For this review, take the finished solid that the model builds, in its own axes (mm). Face numbers are marked on the shaded views. A direction names the side the tool comes from. Give positions to 0.01 mm unless a question says otherwise; leave off trailing zeros. Order: outer loops, then holes, each group sorted by start corner. A loop starts at its lowest first (then second) coordinate and runs counter-clockwise, first axis right, second up. Notation, with made-up numbers: (-5, -27.5) - (26, -27.5) arc R22 ccw to (26, 1.5) - close; hole circle Ø11 at (-35, 40). An arc over 180 degrees is marked (long way). Use a Markdown table: item, result. Add a question column.
1) We need section C-C on y = 113. Write out the cut boundary in (x, z), then the cut area to 3 significant figures.
2) We need section B-B on y = 121.5. Write out the cut boundary in (x, z), then the cut area to 3 significant figures.
3) Wall thickness on L1, parallel to Z at x = -30.25, y = 115.5; L2, parallel to Z at x = -24.5, y = 112.5; L3, parallel to X at y = 127.25, z = 3: over which ranges is each line inside the solid? List them lowest first.
4) Clearance check with flat-ended pins moving along their axes: P1, Ø0.6, axis at y = 116, z = 2.5, coming from the +X side; P2, Ø1, axis at x = -31.5, y = 115, coming from the +Z side; P3, Ø1, axis at x = -23.5, z = 3, coming from the -Y side; P4, Ø3, axis at x = -32, y = 126.5, coming from the -Z side. State where each tip first meets the part, or that it passes through.
5) Machinability: for the marked faces 1, 2 and 3, which of the approach directions +Z, -Z, +X, -X, +Y, -Y give a long, thin tool a straight path to every point of the face, cutting with its end or side? Answer none if there is none.
6) We need section A-A on x = -33.25. Write out the cut boundary in (y, z), then the cut area to 3 significant figures.
7) We need section D-D on x = -27. Write out the cut boundary in (y, z) (3 decimals).
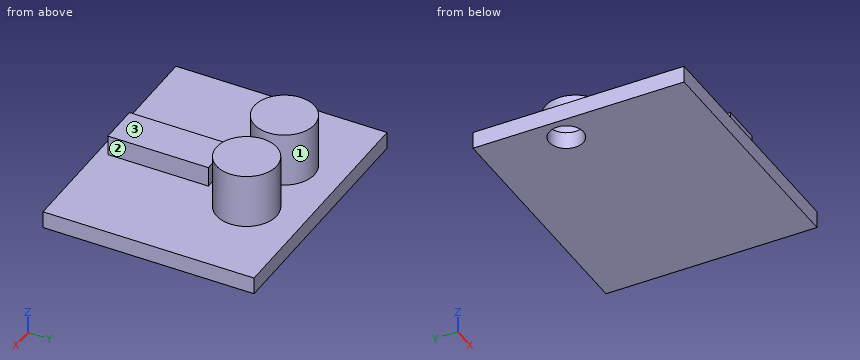
```python
from build123d import *

# Parameters (mm, degrees)
SKETCH_1_W      = 24.7
SKETCH_1_H      = 21
SKETCH_1_R      = 1.7
EXTRUDE_1_DEPTH = 1.7
SKETCH_2_R      = 3
EXTRUDE_2_DEPTH = 5.4
SKETCH_3_W      = 4
SKETCH_3_H      = 10
EXTRUDE_3_DEPTH = 2


with BuildPart() as part:
    # Эскиз1 → Бобышка-Вытянуть1 (new body)
    with BuildSketch(Plane.XY):
        with Locations((-24.007558734, 119.994849308)):
            Rectangle(SKETCH_1_W, SKETCH_1_H)
        with Locations((-33.957558734, 122.494849308)):
            Circle(SKETCH_1_R, mode=Mode.SUBTRACT)
    extrude(amount=EXTRUDE_1_DEPTH)

    # Эскиз2 → Бобышка-Вытянуть2 (add)
    with BuildSketch(Plane.XY.offset(1.7)):
        with Locations(Location((-27.825017342, 124.86066732, 0), (0, 0, 180))):
            Circle(SKETCH_2_R)
        with Locations(Location((-20.796714073, 124.86066732, 0), (0, 0, 180))):
            Circle(SKETCH_2_R)
    extrude(amount=EXTRUDE_2_DEPTH)

    # Эскиз3 → Бобышка-Вытянуть3 (add)
    with BuildSketch(Plane.XY.offset(1.7)):
        with Locations((-23.892041325, 115.47395964)):
            Rectangle(SKETCH_3_W, SKETCH_3_H)
    extrude(amount=EXTRUDE_3_DEPTH)


solid = part.part
```
Checked values:
| question | item | result |
|---|---|---|
| 1 | outline | (-36.36, 0) - (-11.66, 0) - (-11.66, 1.7) - (-21.89, 1.7) - (-21.89, 3.7) - (-25.89, 3.7) - (-25.89, 1.7) - (-36.36, 1.7) - close |
| 1 | area | 50.0 mm² |
| 2 | outline | (-36.36, 0) - (-35.34, 0) - (-35.34, 1.7) - (-36.36, 1.7) - close; (-32.58, 0) - (-11.66, 0) - (-11.66, 1.7) - (-32.58, 1.7) - close |
| 2 | area | 37.3 mm² |
| 3 | L1 | 0 to 1.7 |
| 3 | L2 | 0 to 3.7 |
| 3 | L3 | -29.64 to -26.01, -22.61 to -18.98 |
| 4 | P1 | x = -21.89 |
| 4 | P2 | z = 1.7 |
| 4 | P3 | y = 110.47 |
| 4 | P4 | z = 0 |
| 5 | face 1 | +Z |
| 5 | face 2 | +Z, +X, -Y |
| 5 | face 3 | +Z, +X, -X, -Y |
| 6 | outline | (109.49, 0) - (120.95, 0) - (120.95, 1.7) - (109.49, 1.7) - close; (124.04, 0) - (130.49, 0) - (130.49, 1.7) - (124.04, 1.7) - close |
| 6 | area | 30.4 mm² |
| 7 | outline | (109.495, 0) - (130.495, 0) - (130.495, 1.7) - (127.745, 1.7) - (127.745, 7.1) - (121.976, 7.1) - (121.976, 1.7) - (109.495, 1.7) - close |
